Drawing for the job (mm, zero at the part's lowest x, y, z). Coordinates: 2 decimals unless noted, no trailing zeros. Loops run counter-clockwise (first coordinate to the right, second up) from the corner with the lowest first, then second, coordinate; pieces in that order, holes last. Notation, with made-up numbers: (-25, 81) - (16, 81) arc R11 cw to (16, 99) - close; hole circle Ø9 at (4, 58.5). An arc over 180 degrees is marked (long way). One line per item, written item: value.
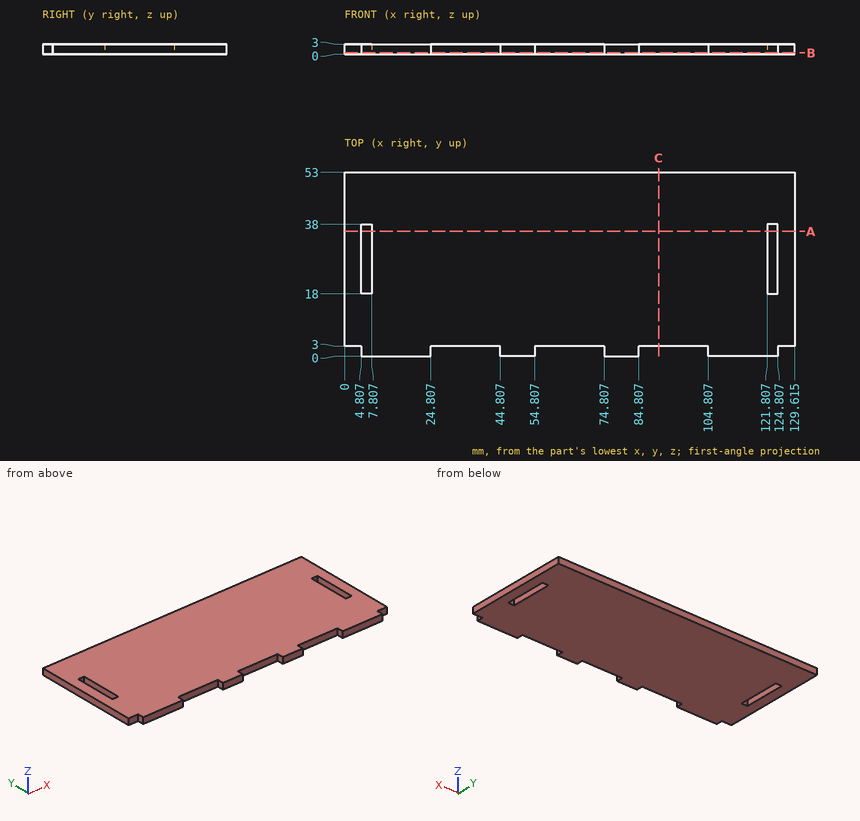
Item 1: Cut at C-C, the plane x = 90.5. Write the cut outline in (y, z), then the cut area to 3 significant figures.
Check result:
outline: (3, 0) - (53, 0) - (53, 3) - (3, 3) - close
area: 150 mm^2
Item 2: Cut at B-B, the plane z = 0.45. Write the cut outline in (x, y) (1 decimal), then the cut area to 3 significant figures.
Check result:
outline: (0, 3) - (4.8, 3) - (4.8, 0) - (24.8, 0) - (24.8, 3) - (44.8, 3) - (44.8, 0) - (54.8, 0) - (54.8, 3) - (74.8, 3) - (74.8, 0) - (84.8, 0) - (84.8, 3) - (104.8, 3) - (104.8, 0) - (124.8, 0) - (124.8, 3) - (129.6, 3) - (129.6, 53) - (0, 53) - close; hole (4.8, 18) - (7.8, 18) - (7.8, 38) - (4.8, 38) - close; hole (121.8, 18) - (124.8, 18) - (124.8, 38) - (121.8, 38) - close
area: 6,540 mm^2
Item 3: Probe probe 1 along X at (y, z) = (26.5, 1.95) (1 decimal); probe 2 along Y at (x, z) = (98, 2.5). List the from-to ranges inside material, lowest first. Write a range as from..to.
Check result:
probe 1: x = 0..4.8, 7.8..121.8, 124.8..129.6
probe 2: y = 3..53
Item 4: Drop flat-ended pins along their axis: P1, Ø1.5, axis at x = 62.5, z = 2, coming from the -Y side; P2, Ø0.9, axis at y = 1, z = 1.5, coming from the -X side; P3, Ø0.9, axis at y = 1.5, z = 1, coming from the +X side. Give the stop position or say it passes through.
Check result:
P1: stops at y = 3
P2: stops at x = 4.81
P3: stops at x = 124.81
Item 5: Cut at A-A, the plane y = 36. Write the cut outline in (x, z) (1 decimal), then the cut area to 3 significant figures.
Check result:
outline: (0, 0) - (4.8, 0) - (4.8, 3) - (0, 3) - close; (7.8, 0) - (121.8, 0) - (121.8, 3) - (7.8, 3) - close; (124.8, 0) - (129.6, 0) - (129.6, 3) - (124.8, 3) - close
area: 371 mm^2
